CAD build for the part. Positions are in the model's coordinates, mm. Coordinates: 2 decimals unless noted, no trailing zeros. Order: outer loops, then holes, each group sorted by start corner. A loop starts at its lowest first (then second) coordinate and runs counter-clockwise, first axis right, second up. Notation, with made-up numbers: (71.5, -7) - (76.5, -7) arc R27 ccw to (76.5, 23) - close; hole circle Ø4 at (78.5, 89.25). An arc over 180 degrees is marked (long way). Return JSON: item names as keys, results as strings.
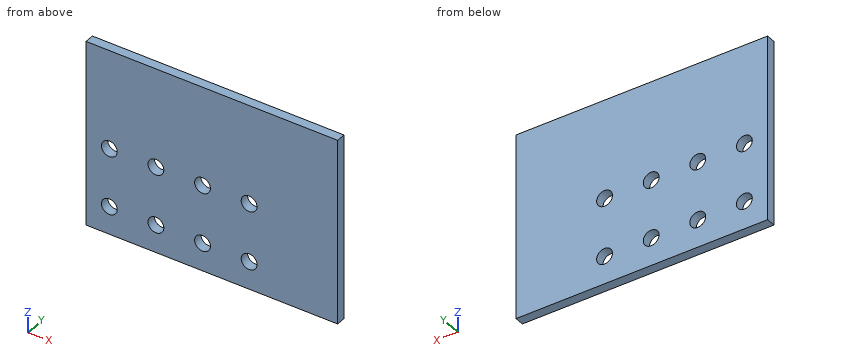
Autodesk Inventor part; units mm, degrees
ref_plane "YZ Plane" through (0, 0, 0) normal (1, 0, 0) x (0, 1, 0)
ref_plane "XZ Plane" through (0, 0, 0) normal (0, 1, 0) x (-1, 0, 0)
ref_plane "XY Plane" through (0, 0, 0) normal (0, 0, 1) x (1, 0, 0)
sketch "Эскиз1" plane through (0, 0, 0) normal (0, 1, 0) x (-1, 0, 0)
  line L0 (-135, -100) -> (135, -100)
  line L1 (135, -100) -> (135, 100)
  line L2 (135, 100) -> (-135, 100)
  line L3 (-135, 100) -> (-135, -100)
  line L4 (-135, -100) -> (135, 100) construction
  line L5 (135, -100) -> (-135, 100) construction
  circle A0 centre (110, -70) radius 8.5
  circle A1 centre (110, -7) radius 8.5
  circle A2 centre (60, -7) radius 8.5
  circle A3 centre (60, -70) radius 8.5
  circle A4 centre (10, -7) radius 8.5
  circle A5 centre (10, -70) radius 8.5
  circle A6 centre (-40, -7) radius 8.5
  circle A7 centre (-40, -70) radius 8.5
  point P0 (0, 0)
  dimension "d0" = 270
  dimension "d1" = 200
  dimension "d2" = 30
  dimension "d3" = 63
  dimension "d4" = 95
  dimension "d5" = 50
  dimension "d6" = 50
  dimension "d7" = 50
  dimension "d8" = 17
extrude "Пластина1" add sketch "Эскиз1" along normal blind 10
equation "\"d6\" = d5"
equation "\"d7\" = d6"
equation "\"d9\" = Толщина"
equation "\"Глубина_просечки\" = 0.5 * Толщина"
properties part number "Lift.03.01.00.02" material "Сталь нержавеющая, 440C"
Item 1: Band-saw the part on A-A, the plane y = 3.25. Count the separate pieces of the cut face and the enclosed holes in it, then the cut area to 3 significant figures.
Findings below:
{"separate pieces": "1", "enclosed holes": "8", "area": "52,200 mm²"}
Item 2: Band-saw the part on C-C, the plane z = -70. List the corners of the cut face in (x, y).
Findings below:
{"outline": "(-135, 0) - (-118.5, 0) - (-118.5, 10) - (-135, 10) - close; (-101.5, 0) - (-68.5, 0) - (-68.5, 10) - (-101.5, 10) - close; (-51.5, 0) - (-18.5, 0) - (-18.5, 10) - (-51.5, 10) - close; (-1.5, 0) - (31.5, 0) - (31.5, 10) - (-1.5, 10) - close; (48.5, 0) - (135, 0) - (135, 10) - (48.5, 10) - close"}
Item 3: Band-saw the part on B-B, the plane x = -10. List the corners of the cut face in (y, z).
Findings below:
{"outline": "(0, -100) - (10, -100) - (10, -78.5) - (0, -78.5) - close; (0, -61.5) - (10, -61.5) - (10, -15.5) - (0, -15.5) - close; (0, 1.5) - (10, 1.5) - (10, 100) - (0, 100) - close"}
Item 4: Drop flat-ended pins along their axis: P1, Ø22, axis at x = 40, z = -7, coming from the +Y side; P2, Ø10, axis at x = -10, z = -70, coming from the +Y side. Give the stop position or say it passes through.
Findings below:
{"P1": "stops at y = 10", "P2": "passes through"}
Item 5: Wall check: L1, parallel to Z at x = -10, y = 8.25; L2, parallel to X at y = 5.5, z = -8; L3, parallel to X at y = 9.5, z = -75. Give the ranges that are in metal, low to high. Write a range as [from, to].
Findings below:
{"L1": "z = [-100, -78.5], [-61.5, -15.5], [1.5, 100]", "L2": "x = [-135, -118.44], [-101.56, -68.44], [-51.56, -18.44], [-1.56, 31.56], [48.44, 135]", "L3": "x = [-135, -116.87], [-103.13, -66.87], [-53.13, -16.87], [-3.13, 33.13], [46.87, 135]"}
